Design review of the part shown in the three views and the two pictorial views. Dimensions are in mm from the part's minimum x, y and z. A direction names the side the tool comes from. Round coordinates to 2 decimals unless told otherwise and drop trailing zeros. Loops run counter-clockwise (first coordinate to the right, second up) from the corner with the lowest first, then second, coordinate; pieces in that order, holes last. Notation, with made-up numbers: (61.25, 81.25) -> (114.25, 81.25) arc R8 ccw to (114.25, 86.25) -> close; hole circle Ø2 at (75.25, 34.5). An arc over 180 degrees is marked (long way). Use a Markdown table: item, result. Add a question column.
1) Mouldability with a two-part tool opening along Y and no side actions: class the marked faces 1, 2, 3 and 4 as released by +Y, released by -Y, zero draft, split by the parting line, or undercut.
2) For the marked faces 5, 6 and 7, list the 3-axis set-ups (+Z, -Z, +X, -X, +Y, -Y) from which the entire face can be reached by the end or side of a thin tool; tool diameter is ignored.
3) Wall thickness on probe 1 along Y at (x, z) = (139, 52) (1 decimal); probe 2 along X at (y, z) = (82, 59.5) (1 decimal); probe 3 along Z at (x, y) = (82.5, 4): over which ranges is each line inside the solid? List them lowest first.
4) Consider section A-A on z = 7. Give the boundary of the cut face in (x, y) (1 decimal).
5) Insertion check: pin 1 (3 mm diameter, centred on x = 87, z = 62, fed in from -Y); pin 2 (18 mm diameter, centred on x = 137, z = 15, fed in from -Y); pin 3 (10 mm diameter, centred on x = 48, y = 10, fed in from +Z); pin 4 (12.5 mm diameter, centred on y = 55.5, z = 25.5, fed in from -X) (1 decimal). Each pin has a flat end and moves straight along its axis. Give the tip position at first contact, or say it passes through.
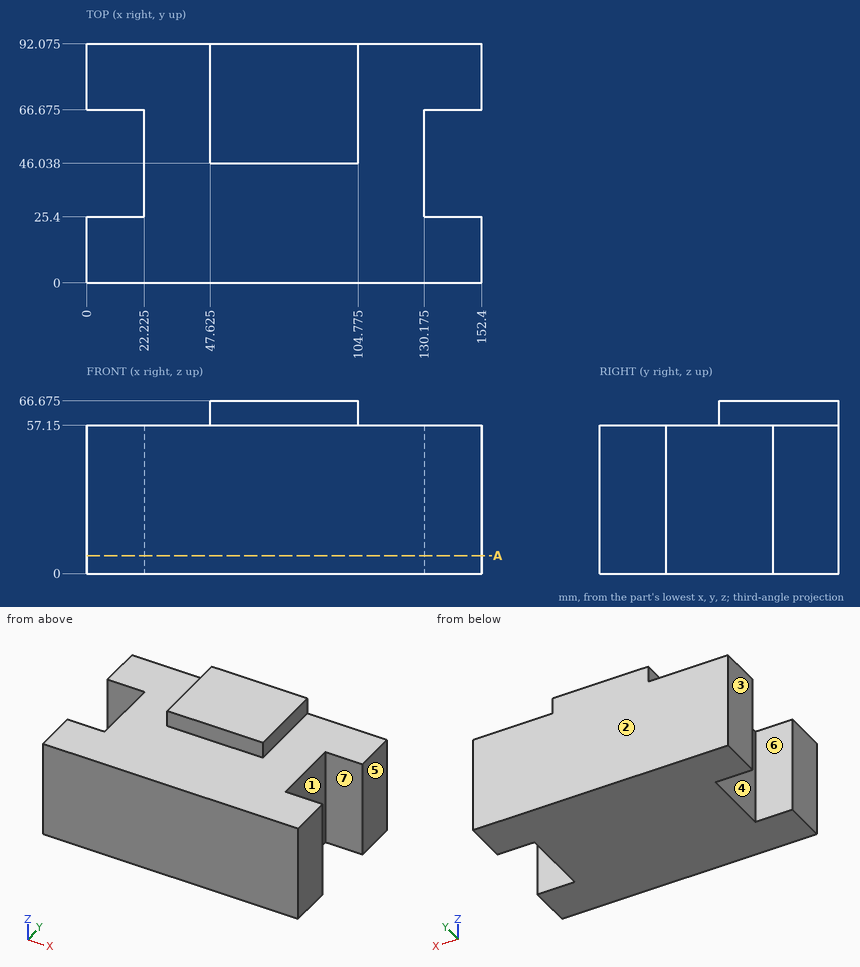
Result set:
| question | item | result |
|---|---|---|
| 1 | face 1 | undercut |
| 1 | face 2 | released by +Y |
| 1 | face 3 | zero draft |
| 1 | face 4 | undercut |
| 2 | face 5 | +Z, -Z, +X, +Y, -Y |
| 2 | face 6 | +Z, -Z, -X |
| 2 | face 7 | +Z, -Z, +X |
| 3 | probe 1 | 0 to 25.4, 66.7 to 92.1 |
| 3 | probe 2 | 47.6 to 104.8 |
| 3 | probe 3 | 0 to 57.15 |
| 4 | outline | (0, 0) -> (152.4, 0) -> (152.4, 25.4) -> (130.2, 25.4) -> (130.2, 66.7) -> (152.4, 66.7) -> (152.4, 92.1) -> (0, 92.1) -> (0, 66.7) -> (22.2, 66.7) -> (22.2, 25.4) -> (0, 25.4) -> close |
| 5 | pin 1 | y = 46.04 |
| 5 | pin 2 | y = 0 |
| 5 | pin 3 | z = 57.15 |
| 5 | pin 4 | x = 22.2 |
